Build history of the part. All positions in model axes, mm. Face numbers are marked on the shaded views. A direction names the side the tool comes from. Round coordinates to 2 decimals unless told otherwise and drop trailing zeros. Write each loop counter-clockwise with the first axis right and the second up, starting at its lowest first coordinate (ties: lowest second). Pieces come first, ordered by that corner, then holes.
1) Saw through at A-A (y = 19.05). Write the cut outline in (x, z), plus the area to 3 significant figures.
2) Saw through at B-B (x = 6.5). Write the cut outline in (y, z).
3) Wall check: probe 1 along X at (y, z) = (19, -2); probe 2 along Z at (x, y) = (0, 4) (3 decimals); probe 3 along Z at (x, y) = (9.75, 23.5). Give the ranges that are in metal, low to high.
4) Flat gauge pins, fed straight in: pin 1 (6 mm diameter, centred on x = 0, y = 53.975, fed in from -Z); pin 2 (5 mm diameter, centred on x = -9.5, z = -31, fed in from +Y). Where does each tip first touch, or does it go through?
5) Saw through at D-D (x = -0.75). Write the cut outline in (y, z).
6) Saw through at C-C (z = -40). Write the cut outline in (x, y).
7) Which spindle directions (+Z, -Z, +X, -X, +Y, -Y) get a long thin tool onto all of the face, cutting with end or side? Do the marked faces 1 and 2. Say none if no direction does.
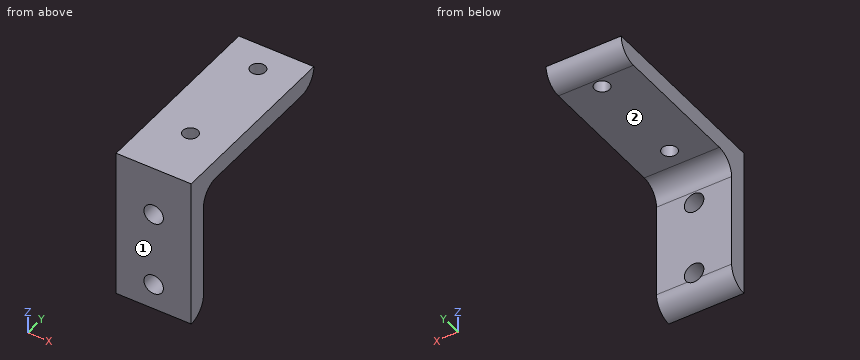
Autodesk Inventor part; units mm, degrees
ref_plane "YZ Plane" through (0, 0, 0) normal (1, 0, 0) x (0, 1, 0)
ref_plane "XZ Plane" through (0, 0, 0) normal (0, 1, 0) x (-1, 0, 0)
ref_plane "XY Plane" through (0, 0, 0) normal (0, 0, 1) x (1, 0, 0)
sketch "Sketch1" plane through (0, 0, 0) normal (1, 0, 0) x (0, 1, 0)
  line L0 (0, 0) -> (63.5, 0)
  line L1 (0, 0) -> (0, -50.8)
  arc A0 (0, -50.8) -> (6.35, -44.45) centre (0, -44.45) ccw
  arc A1 (57.15, -6.35) -> (63.5, 0) centre (57.15, 0) ccw
  line L2 (57.15, -6.35) -> (12.7, -6.35)
  line L3 (6.35, -44.45) -> (6.35, -12.7)
  arc A2 (12.7, -6.35) -> (6.35, -12.7) centre (12.7, -12.7) ccw
  dimension "d0" = 6.35
  dimension "d1" = 63.5
  dimension "d16" = 50.8
extrude "Extrusion1" add sketch "Sketch1" along normal mid plane 25.4
sketch "Sketch2" plane through (-12.7, 0, 0) normal (0, 0, 1) x (1, 0, 0)
  line L0 (25.4, 6.35) -> (0, 6.35)
  line L1 (25.4, 6.35) -> (0, 6.35)
  line L2 (25.4, 6.35) -> (0, 6.35) construction
  line L3 (12.7, 6.35) -> (12.7, 63.5) construction
  line L4 (25.4, 63.5) -> (0, 63.5) construction
  circle A0 centre (12.7, 19.05) radius 2.54
  circle A1 centre (12.7, 53.975) radius 2.54
  point P0 (12.7, 0)
  dimension "d4" = 5.08
  dimension "d5" = 12.7
  dimension "d6" = 9.525
extrude "Extrusion2" cut sketch "Sketch2" against normal through all
sketch "Sketch3" plane through (-12.7, 0, -50.8) normal (0, -1, 0) x (1, 0, 0)
  line L0 (25.4, 44.45) -> (0, 44.45)
  line L1 (25.4, 0) -> (0, 0) construction
  line L2 (12.7, 0) -> (12.7, 44.45) construction
  circle A0 centre (12.7, 34.163) radius 3.302
  circle A1 centre (12.7, 8.763) radius 3.302
  point P0 (12.7, 50.8)
  dimension "d9" = 6.604
  dimension "d14" = 16.637
  dimension "d15" = 25.4
extrude "Extrusion3" cut sketch "Sketch3" against normal through all
properties part number "support L" material "Aluminum 6061"
Evaluation:
1. outline: (-12.7, -6.35) - (-2.54, -6.35) - (-2.54, 0) - (-12.7, 0) - close; (2.54, -6.35) - (12.7, -6.35) - (12.7, 0) - (2.54, 0) - close
1. area: 129 mm2
2. outline: (0, -50.8) arc R6.35 ccw to (6.35, -44.45) - (6.35, -12.7) arc R6.35 cw to (12.7, -6.35) - (57.15, -6.35) arc R6.35 ccw to (63.5, 0) - (0, 0) - close
3. probe 1: x = -12.7 to -2.54, 2.54 to 12.7
3. probe 2: z = -49.382 to -45.339, -38.735 to -19.939, -13.335 to 0
3. probe 3: z = -6.35 to 0
4. pin 1: stops at z = -6.35
4. pin 2: stops at y = 6.35
5. outline: (0, -50.8) arc R6.35 ccw to (6.3, -45.25) - (0, -45.25) - close; (0, -38.82) - (6.35, -38.82) - (6.35, -19.85) - (0, -19.85) - close; (0, -13.42) - (6.35, -13.42) - (6.35, -12.7) arc R6.35 cw to (12.7, -6.35) - (16.62, -6.35) - (16.62, 0) - (0, 0) - close; (21.48, -6.35) - (51.55, -6.35) - (51.55, 0) - (21.48, 0) - close; (56.4, -6.35) - (57.15, -6.35) arc R6.35 ccw to (63.5, 0) - (56.4, 0) - close
6. outline: (-12.7, 0) - (-2.6, 0) - (-2.6, 6.35) - (-12.7, 6.35) - close; (2.6, 0) - (12.7, 0) - (12.7, 6.35) - (2.6, 6.35) - close
7. face 1: +Z, -Z, +X, -X, -Y
7. face 2: -Z, +X, -X, +Y
